Check sheet for the drawn part. Datum: minimum x, y, z corner. Units: mm. A direction names the side the tool comes from. Round coordinates to 2 decimals unless told otherwise and drop trailing zeros. Write each loop counter-clockwise with the first axis right and the second up, starting at its lowest first coordinate (ties: lowest second). Pieces come first, ordered by that corner, then holes.
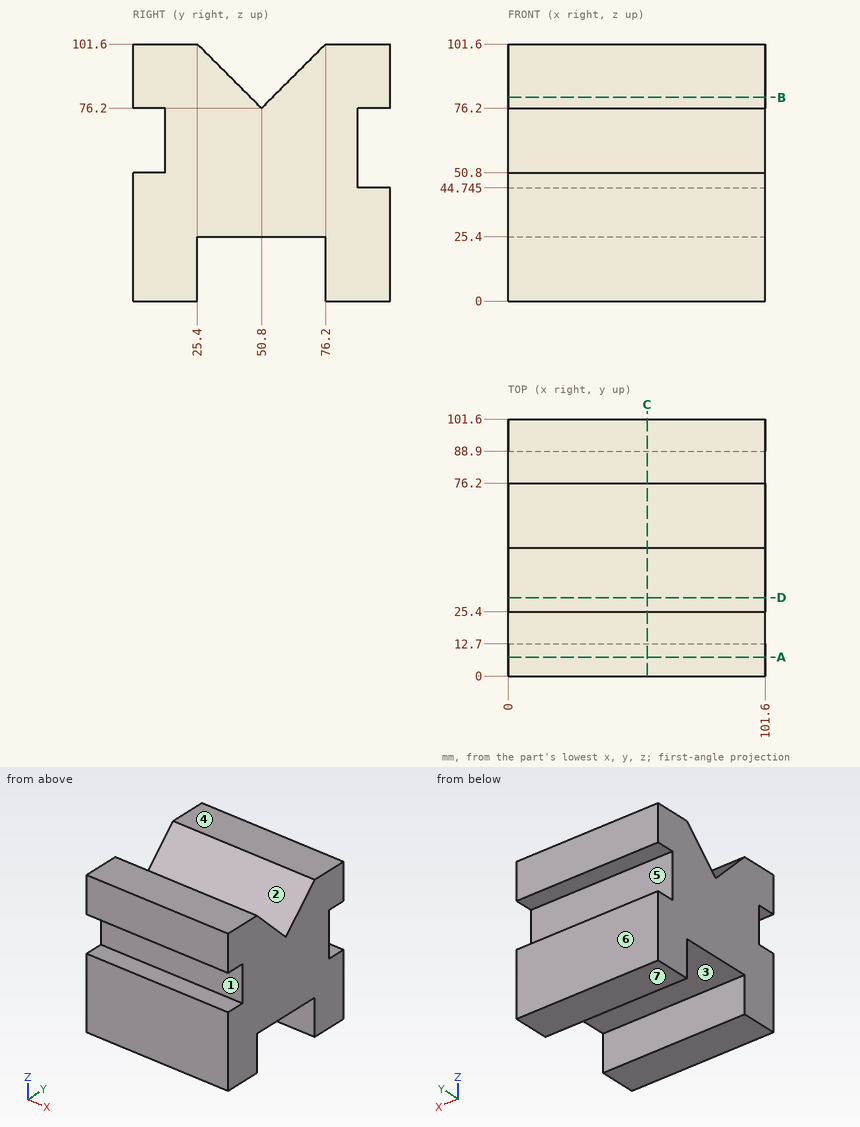
Q1. Material ranges on line 1 along Y through (x, z) = (89, 12); line 2 along Z through (x, y) = (18, 7.5); line 3 along Y through (x, z) = (7.5, 46.5), recorded low to high.
Recorded:
line 1: y = 0 to 25.4, 76.2 to 101.6
line 2: z = 0 to 50.8, 76.2 to 101.6
line 3: y = 0 to 88.9
Q2. Sectioned sample at B-B (z = 80.5). Enter the section's corners in (x, y), plus the area to 3 significant figures.
Recorded:
outline: (0, 0) - (101.6, 0) - (101.6, 46.5) - (0, 46.5) - close; (0, 55.1) - (101.6, 55.1) - (101.6, 101.6) - (0, 101.6) - close
area: 9,450 mm2
Q3. Sectioned sample at D-D (y = 31). Enter the section's corners in (x, z).
Recorded:
outline: (0, 25.4) - (101.6, 25.4) - (101.6, 96) - (0, 96) - close
Q4. Tool access check on the marked faces 1, 2 and 3. Record the directions out of +Z, -Z, +X, -X, +Y, -Y that give a thin tool (end or side, any length) a straight path to the whole face; none if there is none.
Recorded:
face 1: +X, -X, -Y
face 2: +Z, +X, -X
face 3: -Z, +X, -X
Q5. Release check for a two-part mould opening along Z. For the marked faces 4, 5, 6 and 7 record: released by +Z, released by -Z, zero draft, split by the parting line, or undercut.
Recorded:
face 4: released by +Z
face 5: undercut
face 6: zero draft
face 7: released by -Z
Q6. Sectioned sample at A-A (y = 7.5). Enter the section's corners in (x, z), plus the area to 3 significant figures.
Recorded:
outline: (0, 0) - (101.6, 0) - (101.6, 50.8) - (0, 50.8) - close; (0, 76.2) - (101.6, 76.2) - (101.6, 101.6) - (0, 101.6) - close
area: 7,740 mm2
Q7. Depth check by flat-ended pin: P1, Ø1.5, axis at x = 40.5, y = 49, coming from the -Z side; P2, Ø1.5, axis at x = 70.5, y = 30.5, coming from the +Z side; P3, Ø10, axis at x = 20.5, z = 70, coming from the +Y side. Enter the tip coordinate at first touch or a pass-through.
Recorded:
P1: stops at z = 25.4
P2: stops at z = 97.25
P3: stops at y = 88.9
Q8. Sectioned sample at C-C (x = 55). Enter the section's corners in (y, z) (3 decimals).
Recorded:
outline: (0, 0) - (25.4, 0) - (25.4, 25.4) - (76.2, 25.4) - (76.2, 0) - (101.6, 0) - (101.6, 44.745) - (88.9, 44.745) - (88.9, 76.2) - (101.6, 76.2) - (101.6, 101.6) - (76.2, 101.6) - (50.8, 76.2) - (25.4, 101.6) - (0, 101.6) - (0, 76.2) - (12.7, 76.2) - (12.7, 50.8) - (0, 50.8) - close
